from build123d import *

# Parameters (mm, degrees)
F0_R     = 42.8133660757
F1_DEPTH = 25
F2_R     = 62.6286647671
F3_DEPTH = 13
F4_R     = 7.2426406871


with BuildPart() as f1:
    # F0 (on Top) → F1 (new body)
    with BuildSketch(Plane.XY):
        Circle(F0_R)
    extrude(amount=F1_DEPTH)

    # F2 (on Top) → F3 (join)
    with BuildSketch(Plane.XY):
        Circle(F2_R)
    extrude(amount=-F3_DEPTH)

    # F4
    f4_edges = [f1.edges().sort_by_distance(p)[0] for p in [
        (-62.628665, 0, 0),
        (-42.813366, 0, 0),
    ]]
    fillet(f4_edges, radius=F4_R)


solid = f1.part
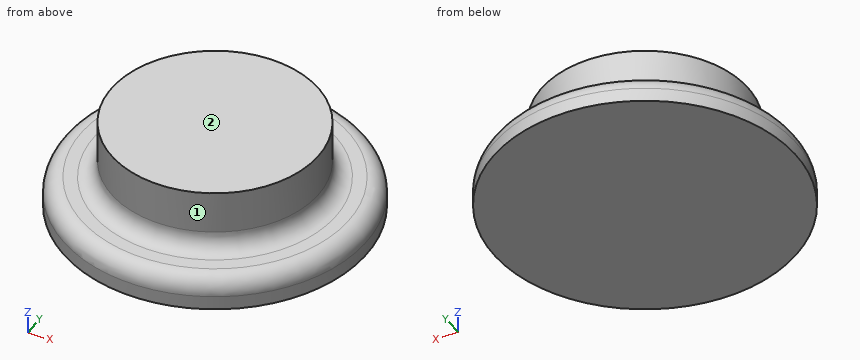
Model file for the job. Use its own axes, mm. Face numbers are marked on the shaded views. A direction names the side the tool comes from. Give positions to 0.01 mm unless a question says otherwise; leave off trailing zeros. Loops run counter-clockwise (first coordinate to the right, second up) from the corner with the lowest first, then second, coordinate; pieces in that order, holes last.
1) Tool access for the marked faces 1 and 2: list every direction of +Z, -Z, +X, -X, +Y, -Y with a clear straight run to the whole face (end or side of a thin tool).
2) Saw through at A-A (x = 0). Write the cut outline in (y, z), plus the area to 3 significant figures.
3) Wall check: line 1 (Z direction, x = -34, y = 43); line 2 (X direction, y = -1, z = -9); line 3 (Y direction, x = 18, z = -2.5). Give the ranges that are in metal, low to high.
4) Saw through at C-C (z = 22). Write the cut outline in (x, y), plus the area to 3 significant figures.
5) Flat gauge pins, fed straight in: pin 1 Ø5 at (y, z) = (-29, -8) entering from +X; pin 2 Ø10 at (y, z) = (-45.5, -3.5) entering from +X; pin 3 Ø2 at (x, z) = (39.5, 16) entering from +Y. Where does each tip first touch, or does it go through?
Answer block:
1. face 1: +Z
1. face 2: +Z, +X, -X, +Y, -Y
2. outline: (-62.63, -13) - (62.63, -13) - (62.63, -7.24) arc R7.24 ccw to (55.39, 0) - (50.06, 0) arc R7.24 cw to (42.81, 7.24) - (42.81, 25) - (-42.81, 25) - (-42.81, 7.24) arc R7.24 cw to (-50.06, 0) - (-55.39, 0) arc R7.24 ccw to (-62.63, -7.24) - close
2. area: 3,770 mm2
3. line 1: z = -13 to 0
3. line 2: x = -62.62 to 62.62
3. line 3: y = -58.14 to 58.14
4. outline: circle Ø85.63 at (0, 0)
4. area: 5,760 mm2
5. pin 1: stops at x = 56.75
5. pin 2: stops at x = 47.14
5. pin 3: stops at y = 18.73
